Design review of the part built by this model. Coordinates are the model's own, in mm. A direction names the side the tool comes from. Give positions to 0.01 mm unless a question says otherwise; leave off trailing zeros. Loops run counter-clockwise (first coordinate to the right, second up) from the corner with the lowest first, then second, coordinate; pieces in that order, holes last. Notation, with made-up numbers: (46, 38.25) - (81, 38.25) arc R11 cw to (81, 58.25) - close; hole circle Ø9 at (-8, 6). An arc over 180 degrees is marked (long way). Write each question's results on one line, items separated by ' | '.
from build123d import *

# Parameters (mm, degrees)
F0_W      = 844.55
F0_H      = 76.2
F1_DEPTH  = 25.4
F2_W      = 12.7
F2_H      = 50.8
F3_DEPTH  = 25.401
F4_W      = 12.7
F4_H      = 6.35
F5_DEPTH  = 76.201
F6_R      = 4.564063
F7_DEPTH  = 50.8
F8_R      = 12.7
F9_DEPTH  = 19.05
F10_W     = 12.7
F10_H     = 19.05
F11_DEPTH = 12.7
F12_W     = 31.75
F12_H     = 25.4
F13_DEPTH = 9.525


with BuildPart() as f1:
    # F0 (on Front) → F1 (new body)
    with BuildSketch(Plane.XZ):
        with Locations((422.275, 38.1)):
            Rectangle(F0_W, F0_H)
    extrude(amount=F1_DEPTH)

    # F2 (on face) → F3 (cut, through all)
    with BuildSketch(Plane.XZ.offset(25.4)):
        with Locations((6.35, 50.8)):
            Rectangle(F2_W, F2_H)
        with Locations((838.2, 50.8)):
            Rectangle(F2_W, F2_H)
    extrude(amount=-F3_DEPTH, mode=Mode.SUBTRACT)

    # F4 (on face) → F5 (cut, through all)
    with BuildSketch(Plane(origin=(0, 0, 0), x_dir=(1, 0, 0), z_dir=(0, 0, -1))):
        with Locations((838.2, 22.225)):
            Rectangle(F4_W, F4_H)
        with Locations((838.2, 3.175)):
            Rectangle(F4_W, F4_H)
        with Locations((6.35, 22.225)):
            Rectangle(F4_W, F4_H)
        with Locations((6.35, 3.175)):
            Rectangle(F4_W, F4_H)
    extrude(amount=-F5_DEPTH, mode=Mode.SUBTRACT)

    # F6 (on face) → F7 (cut)
    with BuildSketch(Plane(origin=(12.7, 0, 0), x_dir=(0, -1, 0), z_dir=(-1, 0, 0))):
        with Locations((12.7, 50.8)):
            Circle(F6_R)
    extrude(amount=-F7_DEPTH, mode=Mode.SUBTRACT)

    # F8 (on face) → F9 (cut)
    with BuildSketch(Plane(origin=(0, 0, 0), x_dir=(-1, 0, 0), z_dir=(0, 1, 0))):
        with Locations((-66.675, 50.8)):
            Circle(F8_R)
        with Locations((-777.875, 50.8)):
            Circle(F8_R)
    extrude(amount=-F9_DEPTH, mode=Mode.SUBTRACT)

    # F10 (on face) → F11 (join)
    with BuildSketch(Plane(origin=(0, 0, 0), x_dir=(-1, 0, 0), z_dir=(0, 1, 0))):
        Polygon((-777.875, 38.1), (-831.85, 38.1), (-831.85, 19.05), (-12.7, 19.05), (-12.7, 38.1), (-66.675, 38.1), align=None)
        with Locations((-838.2, 28.575)):
            Rectangle(F10_W, F10_H)
        with Locations((-6.35, 28.575)):
            Rectangle(F10_W, F10_H)
    extrude(amount=F11_DEPTH)

    # F12 (on face) → F13 (cut)
    with BuildSketch(Plane.XY.offset(76.2)):
        with Locations((228.6, -12.7)):
            Rectangle(F12_W, F12_H)
        with Locations((615.95, -12.7)):
            Rectangle(F12_W, F12_H)
    extrude(amount=-F13_DEPTH, mode=Mode.SUBTRACT)


solid = f1.part
(1) Take a section at A-A on x = 333. Give the boundary of the cut face in (y, z).
Answers below:
outline: (-25.4, 0) - (0, 0) - (0, 19.05) - (12.7, 19.05) - (12.7, 38.1) - (0, 38.1) - (0, 76.2) - (-25.4, 76.2) - close
(2) Draft analysis for pull direction Z (two halves, no side actions). For faces 4 (the flat face through (67, -19.05, 51)), 5 (the flat face through (730, -13, 76.2)), 6 (the flat face through (416, -13, 0)), state which applies: pulls with the +Z half, pulls with the -Z half, needs draft (parallel to the pull), parting line crosses it, or undercut.
Answers below:
face 4: undercut | face 5: pulls with the +Z half | face 6: pulls with the -Z half
(3) Wall thickness on line 1 along X through (y, z) = (-13, 50); line 2 along Z through (x, y) = (41, -12); line 3 along X through (y, z) = (-9.75, 50.8) (3 decimals): over which ranges is each line inside the solid? List them lowest first. Write a range as from..to.
Answers below:
line 1: 79.35..765.2, 790.55..831.85 | line 2: 0..46.29, 55.31..76.2 | line 3: 79.375..765.175, 790.575..831.85
(4) Insertion check: P1, Ø4, axis at x = 388, y = 6, coming from the +Z side; P2, Ø10, axis at x = 841, y = -10, coming from the +Z side; P3, Ø3, axis at y = -13.5, z = 73.5, coming from the +X side. Each pin has a flat end and moves straight along its axis. Give the tip position at first contact, or say it passes through.
Answers below:
P1: z = 38.1 | P2: z = 25.4 | P3: x = 831.85
(5) Tool access review of faces 1 (the flat face through (778, -19.05, 51)), 2 (the flat face through (616, -13, 66.675)), 3 (the flat face through (417, 0, 10)): name each direction out of +Z, -Z, +X, -X, +Y, -Y from which nothing blocks a thin tool from reaching the whole face with its end or side.
Answers below:
face 1: +Y | face 2: +Z, +Y, -Y | face 3: -Z, +X, -X, +Y
